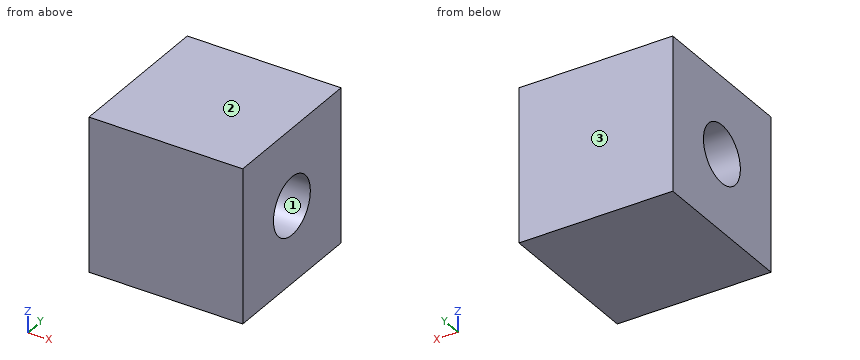
from build123d import *

# Parameters (mm, degrees)
F0_W     = 40
F0_H     = 40
F1_DEPTH = 20
F2_R     = 7.5
F3_DEPTH = 40.001


with BuildPart() as f1:
    # F0 (on Right) → F1 (new body, symmetric)
    with BuildSketch(Plane.YZ):
        Rectangle(F0_W, F0_H)
    extrude(amount=F1_DEPTH, both=True)

    # F2 (on face) → F3 (cut, through all)
    with BuildSketch(Plane.YZ.offset(20)):
        Circle(F2_R)
    extrude(amount=-F3_DEPTH, mode=Mode.SUBTRACT)


solid = f1.part
The listing builds one solid part. Answer for the finished solid, in the listing's coordinates (mm). Face numbers are marked on the shaded views. Round coordinates to 2 decimals unless told otherwise and drop trailing zeros. Order: outer loops, then holes, each group sorted by start corner. A loop starts at its lowest first (then second) coordinate and runs counter-clockwise, first axis right, second up. Notation, with made-up numbers: (-35, 36.25) -> (18, 36.25) arc R12 ccw to (18, 47.25) -> close; hole circle Ø9 at (36, 51). An arc over 180 degrees is marked (long way). Put each result on its own line as item: value.
Q1. Determine the mould class of the marked faces 1, 2 and 3 for opening direction Y: pulls with the +Y half, pulls with the -Y half, needs draft (parallel to the pull), parting line crosses it, or undercut.
Results list:
face 1: undercut
face 2: needs draft
face 3: pulls with the +Y half
Q2. This flat-tipped pin is pushed along its axis until it touches: P1, Ø12, axis at y = 0, z = 0, coming from the -X side. Where does it stop, or does it pass through?
Results list:
P1: through
Q3. Section A-A, the plane y = 0 is taken. Write down the section's boundary in (x, z), and give its area (3 significant figures).
Results list:
outline: (-20, -20) -> (20, -20) -> (20, -7.5) -> (-20, -7.5) -> close; (-20, 7.5) -> (20, 7.5) -> (20, 20) -> (-20, 20) -> close
area: 1,000 mm^2
Q4. Consider line 1 along Z through (x, y) = (-7, 0); line 2 along Z through (x, y) = (-10, 3.5). Determine where each line is inside the solid, lowest interval first.
Results list:
line 1: -20 to -7.5, 7.5 to 20
line 2: -20 to -6.63, 6.63 to 20
Q5. Section C-C, the plane x = -1 is taken. Write down the section's boundary in (y, z).
Results list:
outline: (-20, -20) -> (20, -20) -> (20, 20) -> (-20, 20) -> close; hole circle Ø15 at (0, 0)
